from build123d import *

# Parameters (mm, degrees)
F0_W        = 685.8
F0_H        = 88.9
F0_W_2      = 304.8
F0_H_2      = 19.05
F1_DEPTH    = 38.1
F2_T1_DEPTH = 372.6715659515
F3_R        = 4.2426380505
F4_DEPTH    = 31.75


# Not quite as in the source:
# - a fillet or chamfer that OpenCascade refuses, or shapes differently, is made with other operations: its cross-section is extruded or revolved along the edge and cut away or added


with BuildPart() as f1:
    # F0 (on Top) → F1 (new body)
    with BuildSketch(Plane.XY):
        with Locations((16.0413767457, 5.6168386396)):
            Rectangle(F0_W, F0_H)
        with Locations((-22.0586232543, 5.6168386396)):
            Rectangle(F0_W_2, F0_H_2, mode=Mode.SUBTRACT)
    extrude(amount=F1_DEPTH)

    # F2: fillet of radius 61.3210244843 on 1 edges, made by hand

    # F2_s2 → F2_t1 (cut)
    with BuildSketch(Plane.XZ.offset(-191.9526216153)):
        with BuildLine():
            ThreePointArc((358.9413767457, 0), (336.3654999799, 27.6916706651), (302.1870635554, 38.1))
            Line((302.1870635554, 38.1), (358.9413767457, 38.1))
            Line((358.9413767457, 38.1), (358.9413767457, 0))
        make_face()
    extrude(amount=F2_T1_DEPTH, mode=Mode.SUBTRACT)

    # F3
    f3_edges = [f1.edges().sort_by_distance(p)[0] for p in [
        (358.941377, 5.616839, 0),
    ]]
    fillet(f3_edges, radius=F3_R)

    # F0 (on Top) → F4 (join)
    with BuildSketch(Plane.XY):
        with Locations((-22.0586232543, 5.6168386396)):
            Rectangle(F0_W_2, F0_H_2)
    extrude(amount=F4_DEPTH)


solid = f1.part
Here's how the part is built. I have some questions about the finished solid (model axes, mm). Round coordinates to 2 decimals unless told otherwise and drop trailing zeros. Write each loop counter-clockwise with the first axis right and the second up, starting at its lowest first coordinate (ties: lowest second). Pieces come first, ordered by that corner, then holes.
1. I need wall thicknesses on L1, parallel to X at y = 34, z = 2; L2, parallel to X at y = -25.5, z = 4. Which ranges of each line are inside material? Lowest first, please.
2. Suppose I cut it at B-B (x = 17). List the corners of the cut face in (y, z) for me, and give its area (3 significant figures).
3. Will this pin go through, and if not, where does the flat tip stop? pin 1 Ø3 at (y, z) = (10.5, 11.5) entering from +X.
4. Suppose I cut it at D-D (z = 26). List the corners of the cut face in (x, y) for me, and give its area (3 significant figures).
5. If we mould it in two halves opening along Y, with no side actions, what happens to faces 1 (the flat face through (-17, 16, 38.1)), 2 (the flat face through (10, -38.833, 19)), 3 (the flat face through (-24, 6, 31.75)), 4 (the flat face through (10, 50.067, 19))? For each: released by +Y, released by -Y, zero draft, split by the parting line, or undercut.
6. Suppose I cut it at C-C (y = 35.5). List the corners of the cut face in (x, z) for me, and give its area (3 significant figures).
7. Suppose I cut it at A-A (y = 6.5). List the corners of the cut face in (x, z) for me, and give its area (3 significant figures).
Answer sheet:
1. L1: x = -326.86 to 355.83
1. L2: x = -326.86 to 356.46
2. outline: (-38.83, 0) - (50.07, 0) - (50.07, 38.1) - (15.14, 38.1) - (15.14, 31.75) - (-3.91, 31.75) - (-3.91, 38.1) - (-38.83, 38.1) - close
2. area: 3,270 mm2
3. pin 1: stops at x = 353.73
4. outline: (-326.86, -38.83) - (338.76, -38.83) - (338.76, 50.07) - (-326.86, 50.07) - close
4. area: 59,200 mm2
5. face 1: zero draft
5. face 2: released by -Y
5. face 3: undercut
5. face 4: released by +Y
6. outline: (-326.86, 0) - (352.22, 0) arc R4.24 ccw to (355.94, 6.28) arc R61.32 ccw to (302.19, 38.1) - (-326.86, 38.1) - close
6. area: 25,500 mm2
7. outline: (-326.86, 0) - (352.22, 0) arc R4.24 ccw to (355.94, 6.28) arc R61.32 ccw to (302.19, 38.1) - (130.34, 38.1) - (130.34, 31.75) - (-174.46, 31.75) - (-174.46, 38.1) - (-326.86, 38.1) - close
7. area: 23,600 mm2
